Here's how the part is built. I have some questions about the finished solid (model axes, mm). Face numbers are marked on the shaded views. A direction names the side the tool comes from. Round coordinates to 2 decimals unless told otherwise and drop trailing zeros. Order: outer loops, then holes, each group sorted by start corner. A loop starts at its lowest first (then second) coordinate and runs counter-clockwise, first axis right, second up. Notation, with made-up numbers: (13.5, 3.25) -> (64.5, 3.25) arc R25 cw to (64.5, 41.25) -> close; hole circle Ø5 at (20.25, -20.75). An arc over 180 degrees is marked (long way). Use a Markdown table: item, result. Add a question column.
(1) I want a section at A-A, the plane y = 6.5. Please give me the cut outline in (x, z).
(2) If I drill on probe 1 along X at (y, z) = (4.75, 6); probe 2 along X at (y, z) = (7.5, 3); probe 3 along Y at (x, z) = (21, 1.5), over which ranges is the centre line in solid material (lowest first)?
(3) I want a section at D-D, the plane z = 6. Please give me the cut outline in (x, y).
(4) I'm going to push flat-ended pins straight in: P1, Ø0.9, axis at y = 6.5, z = 3, coming from the +X side; P2, Ø2.5, axis at x = 22.5, z = 2, coming from the +Y side; P3, Ø4, axis at x = 33, z = 3.5, coming from the +Y side. Where does each tip first touch, or does it pass through?
(5) On a 3-axis mill with a long thin cutter (end or side, diameter ignored), from which of +Z, -Z, +X, -X, +Y, -Y can I reach the whole of each face in a straight line? I mean the marked faces 1, 2 and 3. Say none if no direction works.
(6) I want a section at C-C, the plane y = 1.75. Please give me the cut outline in (x, z), then the cut area to 3 significant figures.
(7) I want a section at B-B, the plane x = 5. Please give me the cut outline in (y, z), then the cut area to 3 significant figures.
from build123d import *

# Parameters (mm, degrees)
F1_DEPTH = 2
F2_R     = 1
F4_DEPTH = 8
F5_DEPTH = 5


with BuildPart() as f1:
    # F0 (on Front) → F1 (new body)
    with BuildSketch(Plane.XZ):
        Polygon((0, 3.9), (0, 0), (40, 0), (40, 3.9), (40, 7.8), (20, 7.8), (0, 7.8), align=None)
        with BuildLine():
            ThreePointArc((6.4, 3.9), (5, 2.5), (3.6, 3.9))
            ThreePointArc((3.6, 3.9), (5, 5.3), (6.4, 3.9))
        make_face(mode=Mode.SUBTRACT)
        with BuildLine():
            ThreePointArc((21.4, 3.9), (19.0100505063, 2.9100505063), (20, 5.3))
            ThreePointArc((20, 5.3), (20.9899494937, 4.8899494937), (21.4, 3.9))
        make_face(mode=Mode.SUBTRACT)
        with BuildLine():
            ThreePointArc((33.6, 3.9), (35, 5.3), (36.4, 3.9))
            ThreePointArc((36.4, 3.9), (35, 2.5), (33.6, 3.9))
        make_face(mode=Mode.SUBTRACT)
    extrude(amount=F1_DEPTH)

    # F2
    f2_edges = [f1.edges().sort_by_distance(p)[0] for p in [
        (0, -1, 7.8),
        (0, -1, 0),
        (40, -1, 7.8),
        (40, -1, 0),
    ]]
    fillet(f2_edges, radius=F2_R)

    # F3 (on face) → F4 (join)
    with BuildSketch(Plane(origin=(0, 0, 0), x_dir=(-1, 0, 0), z_dir=(0, 1, 0))):
        Polygon((-13, 7.8), (-13, 3.9), (-13, 0), (-11, 0), (-11, 7.8), align=None)
        Polygon((-27, 0), (-27, 3.9), (-27, 7.8), (-29, 7.8), (-29, 0), align=None)
    extrude(amount=F4_DEPTH)

    # F5 (add): faces of the model
    f5_faces = [f1.faces().sort_by_distance(p)[0] for p in [
        (0.3882451983, 0, 0.3882451983),
        (29.1348480626, 0, 3.9),
    ]]
    extrude(f5_faces, amount=F5_DEPTH)


solid = f1.part
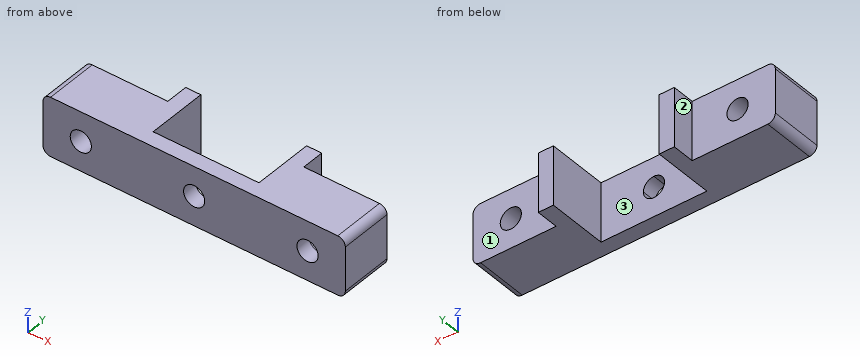
Taken from the geometry:
| question | item | result |
|---|---|---|
| 1 | outline | (11, 0) -> (13, 0) -> (13, 7.8) -> (11, 7.8) -> close; (27, 0) -> (29, 0) -> (29, 7.8) -> (27, 7.8) -> close |
| 2 | probe 1 | x = 0 to 13, 27 to 40 |
| 2 | probe 2 | x = 11 to 13, 27 to 29 |
| 2 | probe 3 | y = -2 to 0 |
| 3 | outline | (0, -2) -> (40, -2) -> (40, 5) -> (29, 5) -> (29, 8) -> (27, 8) -> (27, 0) -> (13, 0) -> (13, 8) -> (11, 8) -> (11, 5) -> (0, 5) -> close |
| 4 | P1 | stops at x = 29 |
| 4 | P2 | stops at y = 0 |
| 4 | P3 | stops at y = 5 |
| 5 | face 1 | +Z, -Z, +X, +Y |
| 5 | face 2 | +Z, -Z, -X, +Y |
| 5 | face 3 | +Z, -Z, +Y |
| 6 | outline | (0, 1) arc R1 ccw to (1, 0) -> (13, 0) -> (13, 7.8) -> (1, 7.8) arc R1 ccw to (0, 6.8) -> close; (27, 0) -> (39, 0) arc R1 ccw to (40, 1) -> (40, 6.8) arc R1 ccw to (39, 7.8) -> (27, 7.8) -> close; hole circle Ø2.8 at (5, 3.9); hole circle Ø2.8 at (35, 3.9) |
| 6 | area | 190 mm2 |
| 7 | outline | (-2, 0) -> (5, 0) -> (5, 2.5) -> (-2, 2.5) -> close; (-2, 5.3) -> (5, 5.3) -> (5, 7.8) -> (-2, 7.8) -> close |
| 7 | area | 35.0 mm2 |
